from build123d import *

# Parameters (mm, degrees)
F0_R      = 127
F1_DEPTH  = 50.8
F2_R      = 88.9
F3_DEPTH  = 1.27
F4_R      = 1.27
F5_DEPTH  = 50.8
F6_R      = 50.8
F7_DEPTH  = 1.27
F8_R      = 88.9
F8_R_2    = 38.1
F9_DEPTH  = 38.1
F10_SIZE  = 7.62
F11_R     = 5.08
F13_DEPTH = 44.45
F14_R     = 30.068591
F14_R_2   = 1.27
F15_DEPTH = 1.27


with BuildPart() as f1:
    # F0 (on Front) → F1 (new body)
    with BuildSketch(Plane.XZ):
        Circle(F0_R)
    extrude(amount=F1_DEPTH)

    # F2 (on face) → F3 (cut)
    with BuildSketch(Plane.XZ.offset(50.8)):
        Circle(F2_R)
    extrude(amount=-F3_DEPTH, mode=Mode.SUBTRACT)

    # F4 (on face) → F5 (cut)
    with BuildSketch(Plane.XZ.offset(49.53)):
        Circle(F4_R)
    extrude(amount=-F5_DEPTH, mode=Mode.SUBTRACT)

    # F6 (on face) → F7 (cut)
    with BuildSketch(Plane.XZ.offset(49.53)):
        Circle(F6_R)
    extrude(amount=-F7_DEPTH, mode=Mode.SUBTRACT)

    # F8 (on face) → F9 (cut)
    with BuildSketch(Plane(origin=(0, 0, 0), x_dir=(-1, 0, 0), z_dir=(0, 1, 0))):
        Circle(F8_R)
        Circle(F8_R_2, mode=Mode.SUBTRACT)
    extrude(amount=-F9_DEPTH, mode=Mode.SUBTRACT)

    # F10
    f10_edges = [f1.edges().sort_by_distance(p)[0] for p in [
        (38.1, -38.1, 0),
    ]]
    chamfer(f10_edges, length=F10_SIZE)

    # F11
    f11_edges = [f1.edges().sort_by_distance(p)[0] for p in [
        (88.9, -38.1, 0),
    ]]
    fillet(f11_edges, radius=F11_R)

    # F12 (on face) → F13 (join)
    with BuildSketch(Plane.XZ.offset(50.8)):
        with BuildLine():
            ThreePointArc((-2.998611, 107.908345), (0, 107.95), (2.998611, 107.908345))
            ThreePointArc((2.998611, 107.908345), (7.602326, 109.70383), (9.525, 114.255894))
            Line((9.525, 114.255894), (9.525, 126.642309))
            ThreePointArc((9.525, 126.642309), (0, 127), (-9.525, 126.642309))
            Line((-9.525, 126.642309), (-9.525, 114.255894))
            ThreePointArc((-9.525, 114.255894), (-7.602326, 109.70383), (-2.998611, 107.908345))
        make_face()
        with BuildLine():
            Line((-74.055926, 87.52631), (-82.814443, 96.284827))
            ThreePointArc((-82.814443, 96.284827), (-89.802561, 89.802561), (-96.284827, 82.814443))
            Line((-96.284827, 82.814443), (-87.52631, 74.055926))
            ThreePointArc((-87.52631, 74.055926), (-82.947979, 72.196666), (-78.42306, 74.182384))
            ThreePointArc((-78.42306, 74.182384), (-76.332177, 76.332177), (-74.182384, 78.42306))
            ThreePointArc((-74.182384, 78.42306), (-72.196666, 82.947979), (-74.055926, 87.52631))
        make_face()
        with BuildLine():
            Line((-114.255894, 9.525), (-126.642309, 9.525))
            ThreePointArc((-126.642309, 9.525), (-127, 0), (-126.642309, -9.525))
            Line((-126.642309, -9.525), (-114.255894, -9.525))
            ThreePointArc((-114.255894, -9.525), (-109.70383, -7.602326), (-107.908345, -2.998611))
            ThreePointArc((-107.908345, -2.998611), (-107.95, 0), (-107.908345, 2.998611))
            ThreePointArc((-107.908345, 2.998611), (-109.70383, 7.602326), (-114.255894, 9.525))
        make_face()
        with BuildLine():
            Line((-87.52631, -74.055926), (-96.284827, -82.814443))
            ThreePointArc((-96.284827, -82.814443), (-89.802561, -89.802561), (-82.814443, -96.284827))
            Line((-82.814443, -96.284827), (-74.055926, -87.52631))
            ThreePointArc((-74.055926, -87.52631), (-72.196666, -82.947979), (-74.182384, -78.42306))
            ThreePointArc((-74.182384, -78.42306), (-76.332177, -76.332177), (-78.42306, -74.182384))
            ThreePointArc((-78.42306, -74.182384), (-82.947979, -72.196666), (-87.52631, -74.055926))
        make_face()
        with BuildLine():
            Line((-9.525, -114.255894), (-9.525, -126.642309))
            ThreePointArc((-9.525, -126.642309), (0, -127), (9.525, -126.642309))
            Line((9.525, -126.642309), (9.525, -114.255894))
            ThreePointArc((9.525, -114.255894), (7.602326, -109.70383), (2.998611, -107.908345))
            ThreePointArc((2.998611, -107.908345), (0, -107.95), (-2.998611, -107.908345))
            ThreePointArc((-2.998611, -107.908345), (-7.602326, -109.70383), (-9.525, -114.255894))
        make_face()
        with BuildLine():
            Line((74.055926, -87.52631), (82.814443, -96.284827))
            ThreePointArc((82.814443, -96.284827), (89.802561, -89.802561), (96.284827, -82.814443))
            Line((96.284827, -82.814443), (87.52631, -74.055926))
            ThreePointArc((87.52631, -74.055926), (82.947979, -72.196666), (78.42306, -74.182384))
            ThreePointArc((78.42306, -74.182384), (76.332177, -76.332177), (74.182384, -78.42306))
            ThreePointArc((74.182384, -78.42306), (72.196666, -82.947979), (74.055926, -87.52631))
        make_face()
        with BuildLine():
            Line((114.255894, -9.525), (126.642309, -9.525))
            ThreePointArc((126.642309, -9.525), (127, 0), (126.642309, 9.525))
            Line((126.642309, 9.525), (114.255894, 9.525))
            ThreePointArc((114.255894, 9.525), (109.70383, 7.602326), (107.908345, 2.998611))
            ThreePointArc((107.908345, 2.998611), (107.95, 0), (107.908345, -2.998611))
            ThreePointArc((107.908345, -2.998611), (109.70383, -7.602326), (114.255894, -9.525))
        make_face()
        with BuildLine():
            Line((87.52631, 74.055926), (96.284827, 82.814443))
            ThreePointArc((96.284827, 82.814443), (89.802561, 89.802561), (82.814443, 96.284827))
            Line((82.814443, 96.284827), (74.055926, 87.52631))
            ThreePointArc((74.055926, 87.52631), (72.196666, 82.947979), (74.182384, 78.42306))
            ThreePointArc((74.182384, 78.42306), (76.332177, 76.332177), (78.42306, 74.182384))
            ThreePointArc((78.42306, 74.182384), (82.947979, 72.196666), (87.52631, 74.055926))
        make_face()
    extrude(amount=-F13_DEPTH)

    # F14 (on face) → F15 (cut)
    with BuildSketch(Plane(origin=(0, 0, 0), x_dir=(-1, 0, 0), z_dir=(0, 1, 0))):
        Circle(F14_R)
        Circle(F14_R_2, mode=Mode.SUBTRACT)
    extrude(amount=-F15_DEPTH, mode=Mode.SUBTRACT)


solid = f1.part
Can you work these out from the model? Positions are in its coordinate system, mm. A direction names the side the tool comes from. Give positions to 0.01 mm unless a question says otherwise; leave off trailing zeros. Answer in a Markdown table with one row per item. Add a question column.
Item 1: We'd pull the mould along Z, two halves only. Please class faces 4 (the flat face through (11, -48.26, 1)), 5 (the cylindrical face through (23.86, -0.63, -18.3)), 6 (the flat face through (26, -50.8, 86)), 7 (the cylindrical face through (0, -29, 127)): released by +Z, released by -Z, zero draft, split by the parting line, or undercut.
Item 2: Please list where these lines run through material, in increasing order: L1, parallel to Z at x = 0, y = -50.1; L2, parallel to Z at x = 0, y = -48; L3, parallel to Z at x = -19, y = -17.
Item 3: For pin 1 Ø1 at (x, y) = (-27, -43.5) entering from -Z; pin 2 Ø4 at (x, y) = (29, -27) entering from +Z; pin 3 Ø12 at (x, y) = (52.5, -10) entering from -Z; pin 4 Ø1.5 at (x, z) = (0, 0) entering from -Y, each with a flat end and sliding along its axis, tell me the tip position at first contact or that it passes through.
Item 4: On a 3-axis mill with a long thin cutter (end or side, diameter ignored), from which of +Z, -Z, +X, -X, +Y, -Y can I reach the whole of each face in a straight line? I mean faces 1 (the flat face through (28, 0, 11.5)), 2 (the flat face through (-6, -1.27, 0)), 3 (the flat face through (38, -49.53, -38)). Say none if no direction works.
Evaluation:
| question | item | result |
|---|---|---|
| 1 | face 4 | undercut |
| 1 | face 5 | undercut |
| 1 | face 6 | zero draft |
| 1 | face 7 | released by +Z |
| 2 | L1 | z = -127 to -88.9, 88.9 to 127 |
| 2 | L2 | z = -127 to -1.27, 1.27 to 127 |
| 2 | L3 | z = -125.57 to -86.85, -33.02 to 33.02, 86.85 to 125.57 |
| 3 | pin 1 | stops at z = -124.2 |
| 3 | pin 2 | stops at z = 124.1 |
| 3 | pin 3 | stops at z = -118.18 |
| 3 | pin 4 | passes through |
| 4 | face 1 | +Z, -Z, +X, -X, +Y |
| 4 | face 2 | +Y |
| 4 | face 3 | -Y |
